The listing builds one solid part. Answer for the finished solid, in the listing's coordinates (mm). Face numbers are marked on the shaded views. A direction names the side the tool comes from. Coordinates: 2 decimals unless noted, no trailing zeros. Order: outer loops, then holes, each group sorted by start corner. A loop starts at its lowest first (then second) coordinate and runs counter-clockwise, first axis right, second up. Notation, with made-up numbers: (86.5, 13) -> (107.5, 13) arc R33 cw to (107.5, 51) -> close; hole circle Ø2 at (56.25, 88). An arc over 180 degrees is marked (long way). Write item = value, one per line.
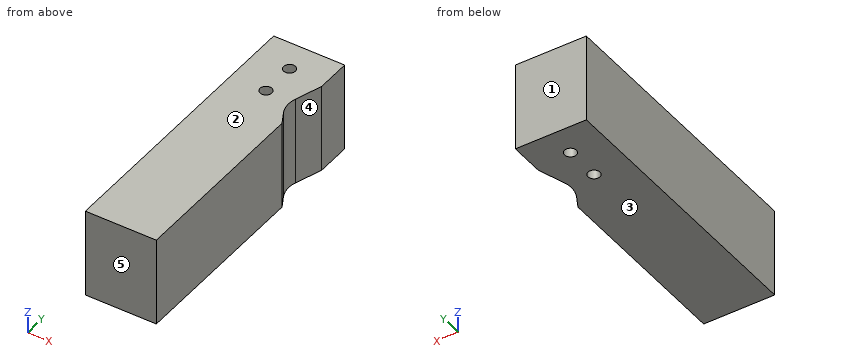
from build123d import *

# Parameters (mm, degrees)
SKETCH1_W           = 19.05
SKETCH1_H           = 76.2
SKETCH1_R           = 1.5875
BOSS_EXTRUDE1_DEPTH = 23.8125
CUT_EXTRUDE1_REACH  = 25.812


with BuildPart() as part:
    # Sketch1 → Boss-Extrude1 (new body)
    with BuildSketch(Plane.XY):
        with Locations((0, -25.4)):
            Rectangle(SKETCH1_W, SKETCH1_H)
        with Locations((0, 4.7625)):
            Circle(SKETCH1_R, mode=Mode.SUBTRACT)
        with Locations((0, -4.7625)):
            Circle(SKETCH1_R, mode=Mode.SUBTRACT)
    extrude(amount=BOSS_EXTRUDE1_DEPTH)

    # Sketch3 → Cut-Extrude1 (cut, up to next)
    with BuildSketch(Plane.XY.offset(23.8125), mode=Mode.PRIVATE) as cut_extrude1_sk1:
        with BuildLine():
            Line((9.525, -12.641309428), (9.525, 3.396941189))
            Line((9.525, 3.396941189), (7.193838245, -3.663696954))
            ThreePointArc((7.193838245, -3.663696954), (6.863457725, -6.55509252), (7.713690054, -9.338332466))
            Line((7.713690054, -9.338332466), (9.525, -12.641309428))
        make_face()
    cut_extrude1_tool1 = extrude(cut_extrude1_sk1.sketch, amount=-CUT_EXTRUDE1_REACH, mode=Mode.PRIVATE) & part.part
    add(cut_extrude1_tool1.solids().sort_by_distance((8.507816, -5.222222, 23.8125))[0], mode=Mode.SUBTRACT)


solid = part.part
Q1. Find the intervals of material crossed by line 1 along Y through (x, z) = (0, 11.5) (3 decimals); line 2 along Y through (x, z) = (-0.5, 3.5); line 3 along X through (y, z) = (-5, 2) (3 decimals), in increasing order.
The answers:
line_1 = -63.5 to -6.35, -3.175 to 3.175, 6.35 to 12.7
line_2 = -63.5 to -6.27, -3.26 to 3.26, 6.27 to 12.7
line_3 = -9.525 to -1.57, 1.57 to 6.891
Q2. A tool of negligible diameter and unlimited length cuts with its end or side. For the marked faces 4 and 5, from which of +Z, -Z, +X, -X, +Y, -Y can it reach the whole face along a straight path? Write none if from no direction.
The answers:
face_4 = +Z, -Z, +X
face_5 = +Z, -Z, +X, -X, -Y
Q3. Section A-A, the plane x = -0.5 is taken. Give the vertices of the cut face in (y, z).
The answers:
outline = (-63.5, 0) -> (-6.27, 0) -> (-6.27, 23.81) -> (-63.5, 23.81) -> close; (-3.26, 0) -> (3.26, 0) -> (3.26, 23.81) -> (-3.26, 23.81) -> close; (6.27, 0) -> (12.7, 0) -> (12.7, 23.81) -> (6.27, 23.81) -> close
Q4. Section B-B, the plane z = 7.75 is taken. Give the vertices of the cut face in (x, y) (1 decimal), plus the area to 3 significant figures.
The answers:
outline = (-9.5, -63.5) -> (9.5, -63.5) -> (9.5, -12.6) -> (7.7, -9.3) arc R7.1 cw to (7.2, -3.7) -> (9.5, 3.4) -> (9.5, 12.7) -> (-9.5, 12.7) -> close; hole circle Ø3.2 at (0, -4.8); hole circle Ø3.2 at (0, 4.8)
area = 1,410 mm2
Q5. The mould has two halves that part along Z. Classify the marked faces 1, 2 and 3: released by +Z, released by -Z, zero draft, split by the parting line, or undercut.
The answers:
face_1 = zero draft
face_2 = released by +Z
face_3 = released by -Z
